For this review, take the finished solid that the model builds, in its own axes (mm). Face numbers are marked on the shaded views. A direction names the side the tool comes from. Give positions to 0.01 mm unless a question says otherwise; leave off trailing zeros. Write each loop counter-clockwise with the first axis right and the second up, starting at its lowest first coordinate (ties: lowest second). Pieces come first, ordered by that corner, then holes. Notation, with made-up numbers: (69.5, 76.5) -> (123.5, 76.5) arc R23 ccw to (123.5, 105.5) -> close; hole circle Ø7 at (62, 38.5). An arc over 180 degrees is marked (long way). Write item = value, one per line.
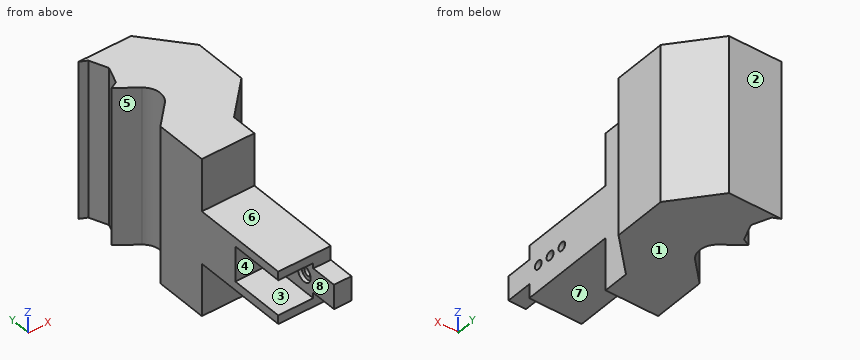
Autodesk Inventor part; units mm, degrees
ref_plane "Work Plane1" through (0, 0, -15) normal (0, 0, 1) x (1, 0, 0)
ref_plane "YZ Plane" through (0, 0, 0) normal (1, 0, 0) x (0, 1, 0)
ref_plane "XZ Plane" through (0, 0, 0) normal (0, 1, 0) x (-1, 0, 0)
sketch "Sketch1" plane through (0, 0, 0) normal (0, 0, 1) x (1, 0, 0)
  line L0 (0, 0) -> (25, 0)
  line L1 (25, 0) -> (25, 40)
  line L2 (25, 40) -> (0, 40)
  line L3 (0, 40) -> (0, 0)
  dimension "d1" = 25
  dimension "d2" = 40
  dimension "d3" = 25
extrude "Extrusion1" add sketch "Sketch1" against normal blind 30
sketch "Sketch2" plane through (25, 0, 0) normal (1, 0, 0) x (0, 0, -1)
  line L0 (0, 0) -> (30, 0)
  circle A0 centre (15, 6.56) radius 2.46
extrude "Extrusion2" cut sketch "Sketch2" against normal blind 30
sketch "Sketch3" plane through (0, 0, 0) normal (-1, 0, 0) x (0, 0, 1)
  line L0 (0, 0) -> (-30, 0)
  line L1 (-25.05, 0) -> (-4.95, 0)
  line L2 (-4.95, 0) -> (-4.95, 33.12)
  line L3 (-4.95, 33.12) -> (-25.05, 33.12)
  line L4 (-25.05, 33.12) -> (-25.05, 0)
  dimension "d11" = 20.1
extrude "Extrusion3" cut sketch "Sketch3" against normal blind 20
sketch "Sketch4" plane through (0, 0, 0) normal (0, -1, 0) x (1, 0, 0)
  line L0 (20, -4.95) -> (20, -25.05)
  line L1 (20, -15) -> (25, -15)
  line L2 (25, 0) -> (25, -30)
  line L3 (20, -8.025) -> (25, -8.025)
  line L4 (25, -8.025) -> (25, -21.975)
  line L5 (25, -21.975) -> (20, -21.975)
  line L6 (20, -21.975) -> (20, -8.025)
  line L7 (20, -8.025) -> (25, -21.975) construction
  line L8 (25, -8.025) -> (20, -21.975) construction
  line L9 (25, -12.54) -> (25, -17.46)
  point P0 (0, 0)
  point P1 (22.5, -15)
  dimension "d14" = 13.95
extrude "Extrusion4" add sketch "Sketch4" along normal blind 15
sketch "Sketch5" plane through (20, 0, 0) normal (-1, 0, 0) x (0, 0, 1)
  circle A0 centre (-15, 6.56) radius 2.46
  circle A1 centre (-15, 6.56) radius 4.7025
  circle A2 centre (-15, 6.56) radius 2.46
  circle A3 centre (-15, 6.56) radius 2.46
  point P0 (0, 0)
  dimension "d17" = 9.405
extrude "Extrusion5" cut sketch "Sketch5" against normal blind 2.1
sketch "Sketch6" plane through (25, 0, 0) normal (1, 0, 0) x (0, 0, -1)
  circle A0 centre (15, 6.56) radius 4.7025
  line L0 (15, 6.56) -> (15, 23.56)
  circle A1 centre (15, 23.56) radius 2.46
  point P0 (0, 0)
  dimension "d20" = 17
  dimension "d21" = 4.92
extrude "Extrusion6" cut sketch "Sketch6" against normal blind 10 contours A1
sketch "Sketch7" plane through (20, 0, 0) normal (-1, 0, 0) x (0, 0, 1)
  circle A0 centre (-15, 23.56) radius 2.46
  circle A1 centre (-15, 23.56) radius 4.7025
  point P0 (0, 0)
  dimension "d24" = 9.405
extrude "Extrusion7" cut sketch "Sketch7" against normal blind 2.1
sketch "Sketch9" plane through (25, 0, 0) normal (1, 0, 0) x (0, 0, -1)
  circle A0 centre (15, 6.56) radius 2.46
  circle A1 centre (15, 6.56) radius 2.46
  circle A2 centre (15, 23.56) radius 2.46
  circle A3 centre (15, 23.56) radius 2.46
  line L0 (30, 40) -> (30, 0)
  line L1 (30, 0) -> (30, 40)
  line L2 (30, 40) -> (0, 40)
  line L3 (0, 40) -> (0, 0)
  line L4 (0, 0) -> (8.025, 0)
  line L5 (21.975, 0) -> (21.975, -15)
  line L6 (21.975, -15) -> (8.025, -15)
  line L7 (8.025, -15) -> (8.025, 0)
  line L8 (0, 0) -> (8.025, 0)
  line L9 (21.975, 0) -> (30, 0)
extrude "Extrusion8" add sketch "Sketch9" along normal blind 5
sketch "Sketch10" plane through (0, 40, 0) normal (0, 1, 0) x (1, 0, 0)
  line L0 (0, 30) -> (30, 30)
  line L1 (30, 0) -> (0, 0)
  line L2 (0, 30) -> (30, 30)
  line L3 (30, 30) -> (30, 0)
  line L4 (30, 0) -> (0, 0)
  line L5 (0, 0) -> (0, 30)
extrude "Extrusion9" add sketch "Sketch10" along normal blind 30
sketch "Sketch12" plane through (30, 0, 0) normal (1, 0, 0) x (0, 0, -1)
  circle A0 centre (15, 6.56) radius 2.46
  line L0 (15, 6.56) -> (15, 15.06)
  circle A1 centre (15, 15.06) radius 2.525
  point P0 (0, 0)
  dimension "d31" = 8.5
  dimension "d33" = 5.05
extrude "Extrusion10" cut sketch "Sketch12" against normal blind 30 contours A1
sketch "Sketch15" plane through (0, 0, -25.05) normal (-1, 0, 0) x (0, 0, 1)
  line L0 (0, 33.12) -> (20.1, 33.12)
  line L1 (20.1, 33.12) -> (20.1, 0)
  line L2 (0, 33.12) -> (20.1, 33.12)
  line L3 (20.1, 33.12) -> (20.1, 31.1)
  line L4 (20.1, 31.1) -> (0, 31.1)
  line L5 (0, 31.1) -> (0, 33.12)
  point P0 (25.05, 0)
  dimension "d57" = 2.02
extrude "Extrusion13" add sketch "Sketch15" against normal blind 20
sketch "Sketch17" plane through (0, 0, 0) normal (0, 0, 1) x (1, 0, 0)
  line L0 (0, 70) -> (30, 70)
  line L1 (30, 70) -> (50.0622, 90.0622)
  line L2 (30, 70) -> (80, 70) construction
  line L3 (11.9522, 97.2454) -> (0, 85.2932)
  line L4 (0, 70) -> (0, 85.2932)
  line L5 (0, 70) -> (0, 0)
  line L6 (0, 70) -> (30, 70)
  line L7 (10.923, 112.2849) -> (0, 120.567)
  line L8 (50.0622, 105.3553) -> (50.0622, 120.567)
  line L9 (50.0622, 105.3553) -> (50.0622, 90.0622)
  arc A0 (11.9522, 97.2454) -> (10.923, 112.2849) centre (4.8811, 104.3165) ccw
  line L10 (0, 144.567) -> (30, 144.567)
  line L11 (30, 144.567) -> (50.0622, 120.567)
  line L12 (4, 142.567) -> (0, 144.567)
  line L13 (4, 122.567) -> (0, 120.567)
  line L14 (4, 122.567) -> (8, 132.567)
  line L15 (8, 132.567) -> (4, 142.567)
  dimension "d61" = 45
  dimension "d62" = 32.0271
  dimension "d72" = 10
extrude "Extrusion14" add sketch "Sketch17" against normal blind 30
sketch "Sketch22" plane through (0, 0, 0) normal (0, 0, 1) x (1, 0, 0)
  line L0 (11.9522, 97.2454) -> (0, 85.2932)
  line L1 (0, 85.2932) -> (11.9522, 97.2454)
  arc A0 (11.9522, 97.2454) -> (10.923, 112.2849) centre (4.8811, 104.3165) ccw
  arc A1 (11.9522, 97.2454) -> (10.923, 112.2849) centre (4.8811, 104.3165) ccw
  line L2 (0, 120.567) -> (10.923, 112.2849)
  line L3 (10.923, 112.2849) -> (0, 120.567)
  line L4 (0, 120.567) -> (4, 122.567)
  line L5 (0, 120.567) -> (4, 122.567)
  line L6 (4, 122.567) -> (8, 132.567)
  line L7 (4, 122.567) -> (8, 132.567)
  line L8 (8, 132.567) -> (4, 142.567)
  line L9 (8, 132.567) -> (4, 142.567)
  line L10 (4, 142.567) -> (0, 144.567)
  line L11 (4, 142.567) -> (0, 144.567)
  line L12 (0, 144.567) -> (30, 144.567)
  line L13 (0, 144.567) -> (30, 144.567)
  line L14 (50.0622, 120.567) -> (30, 144.567)
  line L15 (30, 144.567) -> (50.0622, 120.567)
  line L16 (50.0622, 120.567) -> (50.0622, 90.0622)
  line L17 (50.0622, 120.567) -> (50.0622, 90.0622)
  line L18 (30, 70) -> (50.0622, 90.0622)
  line L19 (50.0622, 90.0622) -> (30, 70)
  line L20 (0, 0) -> (0, 85.2932)
  line L21 (0, 85.2932) -> (0, 55.2932)
  line L22 (0, 55.2932) -> (30, 55.2932)
  line L23 (30, 0) -> (30, 70)
  line L24 (30, 55.2932) -> (30, 70)
  dimension "d83" = 30
extrude "Extrusion15" add sketch "Sketch22" along normal blind 30
ref_plane "Work Plane1" through (0, 0, -15) normal (0, 0, 1) x (1, 0, 0)
mirror "Mirror1" about plane through (0, 0, -15) normal (0, 0, 1) of "Extrusion15"
properties part number "rec_c_20mm_x_90mm"
(1) Take a section at A-A (x = 24.5). Write out the cut boundary in (y, z) (3 decimals).
Answers below:
outline = (-15, -21.975) -> (0, -21.975) -> (0, -30) -> (55.293, -30) -> (55.293, -60) -> (144.567, -60) -> (144.567, 30) -> (55.293, 30) -> (55.293, 0) -> (0, 0) -> (0, -8.025) -> (-15, -8.025) -> close; hole circle Ø4.92 at (6.56, -15); hole circle Ø5.05 at (15.06, -15); hole circle Ø4.92 at (23.56, -15)
(2) Take a section at D-D (z = -15). Count the separate pieces of the cut face and the enclosed holes in it, plus the area to 3 significant figures.
Answers below:
separate_pieces = 4
enclosed_holes = 0
area = 4,300 mm^2
(3) Take a section at C-C (z = -52.5). Write out the cut boundary in (x, y), plus the area to 3 significant figures.
Answers below:
outline = (0, 55.29) -> (30, 55.29) -> (30, 70) -> (50.06, 90.06) -> (50.06, 120.57) -> (30, 144.57) -> (0, 144.57) -> (4, 142.57) -> (8, 132.57) -> (4, 122.57) -> (0, 120.57) -> (10.92, 112.28) arc R10 cw to (11.95, 97.25) -> (0, 85.29) -> close
area = 3,280 mm^2
(4) For pin 1 (2.5 mm diameter, centred on x = 8, z = -3, fed in from -Y); pin 2 (5.5 mm diameter, centred on y = 23.56, z = -15, fed in from -X); pin 3 (11 mm diameter, centred on y = 23.56, z = -15, fed in from -X); pin 4 (3 mm diameter, centred on y = 15.06, z = -15, fed in from -X), all flat-tipped, find the tip position at first contact; note any pin that passes through.
Answers below:
pin_1 = 0
pin_2 = 22.1
pin_3 = 20
pin_4 = through
(5) To check wall thickness, follow probe 1 along Y at (x, z) = (27, -15) (3 decimals); probe 2 along Y at (x, z) = (20.6, -15) (1 decimal); probe 3 along Z at (x, y) = (22, 15). State the ranges of each line that lie inside material, in increasing order.
Answers below:
probe_1 = -15 to 4.1, 9.02 to 12.535, 17.585 to 21.1, 26.02 to 144.567
probe_2 = -15 to 1.9, 11.3 to 12.5, 17.6 to 18.9, 28.3 to 144.6
probe_3 = -30 to -17.52, -12.48 to 0
(6) Tool access review of the marked faces 5, 6, 7 and 8: name each direction out of +Z, -Z, +X, -X, +Y, -Y from which nothing blocks a thin tool from reaching the whole face with its end or side.
Answers below:
face_5 = +Z, -Z, -X
face_6 = +Z, +X, -X, -Y
face_7 = -Z, +X, -X, -Y
face_8 = -X, -Y
(7) Take a section at B-B (y = 6.56). Write out the cut boundary in (x, z).
Answers below:
outline = (0, -30) -> (30, -30) -> (30, -17.46) -> (22.1, -17.46) -> (22.1, -19.7) -> (20, -19.7) -> (20, -25.05) -> (0, -25.05) -> close; (0, -4.95) -> (20, -4.95) -> (20, -10.3) -> (22.1, -10.3) -> (22.1, -12.54) -> (30, -12.54) -> (30, 0) -> (0, 0) -> close
(8) The part is to be moulded in two halves that separate along Z. For the marked faces 1, 2, 3 and 4, say which applies: released by +Z, released by -Z, zero draft, split by the parting line, or undercut.
Answers below:
face_1 = released by -Z
face_2 = zero draft
face_3 = undercut
face_4 = undercut
